Check sheet for the modelled part. Datum: model origin and axes. Units: mm. Round coordinates to 2 decimals unless told otherwise and drop trailing zeros. Write each loop counter-clockwise with the first axis right and the second up, starting at its lowest first coordinate (ties: lowest second). Pieces come first, ordered by that corner, then holes. Notation, with made-up numbers: (73, -19.5) -> (129, -19.5) arc R26 ccw to (129, 4.5) -> close; hole circle Ø3 at (-11.5, 11.25). An arc over 180 degrees is marked (long way). Write item = value, one per line.
from build123d import *

# Parameters (mm, degrees)
SKETCH_1_W             = 0.8
SKETCH_1_H             = 15
EXTRUDE_1_DEPTH        = 203
SKETCH_2_R             = 2.5
SKETCH_3_R             = 1.5
CUT_EXTRUDE_1_DEPTH    = 407.407738607
SKETCH_10_W            = 33
SKETCH_10_H            = 6
SKETCH_10_W_2          = 21.5
CUT_EXTRUDE_4_DEPTH    = 60
PATTERN_LINEAR_1_COUNT = 8
PATTERN_LINEAR_1_PITCH = 50


with BuildPart() as part:
    # 草图1 → 拉伸-薄壁1 (new, symmetric)
    with BuildSketch(Plane.XY):
        with Locations((0.4, 7.5)):
            Rectangle(SKETCH_1_W, SKETCH_1_H)
    extrude(amount=EXTRUDE_1_DEPTH, both=True)

    # 扫描1: sweep along a curve in space
    with BuildLine() as sweep_1_path:
        Line((0.8, 15, 203), (0.8, 15, -203))
    # 草图2 → 扫描1 (sweep)
    with BuildSketch(Plane.XY.offset(203)):
        with Locations((2.5, 15)):
            Circle(SKETCH_2_R)
    sweep(path=sweep_1_path.line)

    # 草图3 → 切除-拉伸1 (cut, through all)
    with BuildSketch(Plane.XY.offset(203)):
        with Locations((2.5, 15)):
            Circle(SKETCH_3_R)
    extrude(amount=-CUT_EXTRUDE_1_DEPTH, mode=Mode.SUBTRACT)

    # 草图10 → 切除-拉伸4 (cut, symmetric)
    with BuildSketch(Plane(origin=(0.8, 0, 0), x_dir=(0, 0, -1), z_dir=(1, 0, 0))):
        with Locations((-132, 15)):
            Rectangle(SKETCH_10_W, SKETCH_10_H)
        with Locations((-192.25, 15)):
            Rectangle(SKETCH_10_W_2, SKETCH_10_H)
        with Locations((-66, 15.006165986)):
            Rectangle(SKETCH_10_W, SKETCH_10_H)
        with Locations((0, 15.012331973)):
            Rectangle(SKETCH_10_W, SKETCH_10_H)
        with Locations((66, 15.018497959)):
            Rectangle(SKETCH_10_W, SKETCH_10_H)
        with Locations((132, 15.024663945)):
            Rectangle(SKETCH_10_W, SKETCH_10_H)
        with Locations((192.25, 15.030829932)):
            Rectangle(SKETCH_10_W_2, SKETCH_10_H)
    extrude(amount=CUT_EXTRUDE_4_DEPTH, both=True, mode=Mode.SUBTRACT)

    # 草图11 → M3 锥坑平头螺钉的锥形沉头孔1 (revolve, cut)
    with BuildSketch(Plane(origin=(0.8, 5.5, -175), x_dir=(0, 0, -1), z_dir=(0, 1, 0))):
        Polygon((0, 0), (0, 0.8), (1.7, 0.8), (1.7, 1.45), (3.15, 0), align=None)
    hole_wizard_m3_1 = revolve(axis=Axis((7.15, 5.5, -175), (-1, 0, 0)), mode=Mode.SUBTRACT)

    # 阵列(线性)1: M3 锥坑平头螺钉的锥形沉头孔1 ×8
    with Locations(*[(0, 0, i * PATTERN_LINEAR_1_PITCH) for i in range(1, PATTERN_LINEAR_1_COUNT)]):
        add(hole_wizard_m3_1, mode=Mode.SUBTRACT)


solid = part.part
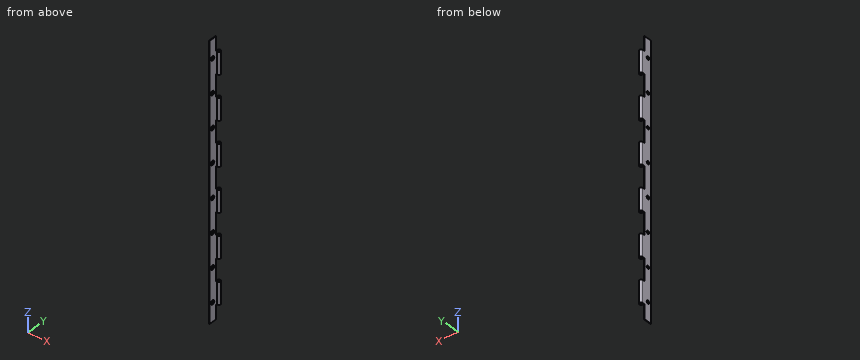
(1) Go/stop test with flat-tipped pins: P1, Ø2.5, axis at x = 1.5, y = 16, coming from the -Z side; P2, Ø3, axis at x = 2, z = 65.5, coming from the +Y side; P3, Ø6.5, axis at y = 6, z = 61.5, coming from the +X side. Record where each tip stops, or that it passes through.
Worked answers:
P1 = -181.5
P2 = 12.01
P3 = 0.8
(2) Sectioned sample at B-B on x = 2.5. Count the separate pieces of the cut face and the enclosed holes in it, then the cut area to 3 significant figures.
Worked answers:
separate_pieces = 12
enclosed_holes = 0
area = 396 mm²
(3) Sectioned sample at C-C on z = -10. Enter the section's corners in (x, y).
Worked answers:
outline = (0, 0) -> (0.8, 0) -> (0.8, 12.01) -> (0, 12.01) -> close
(4) Material ranges on L1, parallel to Z at x = 4.65, y = 15; L2, parallel to Y at x = 2.5, z = 32; L3, parallel to X at y = 6.5, z = -114, recorded low to high. Write a range as [from, to].
Worked answers:
L1 = [-181.5, -148.5], [-115.5, -82.5], [-49.5, -16.5], [16.5, 49.5], [82.5, 115.5], [148.5, 181.5]
L2 = [12.5, 13.5], [16.5, 17.5]
L3 = [0, 0.8]
(5) Sectioned sample at A-A on z = -159. Enter the section's corners in (x, y), then the cut area to 3 significant figures.
Worked answers:
outline = (0, 0) -> (0.8, 0) -> (0.8, 13.17) arc R2.5 ccw (long way) to (0, 15) -> close; hole circle Ø3 at (2.5, 15)
area = 23.6 mm²
